Design review of the part built by this model. Coordinates are the model's own, in mm. Coordinates: 2 decimals unless noted, no trailing zeros. Write each loop counter-clockwise with the first axis right and the second up, starting at its lowest first coordinate (ties: lowest second). Pieces come first, ordered by that corner, then holes. Notation, with made-up numbers: (61, -33) - (103, -33) arc R23 ccw to (103, -6) - close; hole circle Ø3 at (-25, 39.5). An arc over 180 degrees is marked (long way). Use a Markdown table: item, result.
from build123d import *

# Parameters (mm, degrees)
SKETCH1_W           = 25.4
SKETCH1_H           = 50.8
SKETCH1_W_2         = 20.32
SKETCH1_H_2         = 45.72
BOSS_EXTRUDE1_DEPTH = 1314.45
SKETCH2_W           = 25.4
SKETCH2_H           = 50.8
BOSS_EXTRUDE2_DEPTH = 6.35
SKETCH3_W           = 25.4
SKETCH3_H           = 50.8
BOSS_EXTRUDE3_DEPTH = 6.35
SKETCH4_W           = 19.05
SKETCH4_H           = 19.05
SKETCH4_W_2         = 12.7
SKETCH4_H_2         = 12.7
BOSS_EXTRUDE4_DEPTH = 558.8


with BuildPart() as part:
    # Sketch1 → Boss-Extrude1 (new body, symmetric)
    with BuildSketch(Plane(origin=(0, 0, 0), x_dir=(0, 0, -1), z_dir=(1, 0, 0))):
        Rectangle(SKETCH1_W, SKETCH1_H)
        Rectangle(SKETCH1_W_2, SKETCH1_H_2, mode=Mode.SUBTRACT)
    extrude(amount=BOSS_EXTRUDE1_DEPTH, both=True)

    # Sketch2 → Boss-Extrude2 (add)
    with BuildSketch(Plane(origin=(1314.45, 0, 0), x_dir=(0, 0, -1), z_dir=(1, 0, 0))):
        Rectangle(SKETCH2_W, SKETCH2_H)
    extrude(amount=BOSS_EXTRUDE2_DEPTH)

    # Sketch3 → Boss-Extrude3 (add)
    with BuildSketch(Plane.ZY.offset(1314.45)):
        Rectangle(SKETCH3_W, SKETCH3_H)
    extrude(amount=BOSS_EXTRUDE3_DEPTH)

    # Sketch4 → Boss-Extrude4 (add)
    with BuildSketch(Plane(origin=(0, 0, -12.7), x_dir=(-1, 0, 0), z_dir=(0, 0, -1))):
        with Locations((-1282.573, -12.7)):
            Rectangle(SKETCH4_W, SKETCH4_H)
        with Locations((-1282.573, -12.7)):
            Rectangle(SKETCH4_W_2, SKETCH4_H_2, mode=Mode.SUBTRACT)
        with Locations((-508, -12.7)):
            Rectangle(SKETCH4_W, SKETCH4_H)
        with Locations((-508, -12.7)):
            Rectangle(SKETCH4_W_2, SKETCH4_H_2, mode=Mode.SUBTRACT)
        with Locations((1282.573, -12.7)):
            Rectangle(SKETCH4_W, SKETCH4_H)
        with Locations((1282.573, -12.7)):
            Rectangle(SKETCH4_W_2, SKETCH4_H_2, mode=Mode.SUBTRACT)
        with Locations((508, -12.7)):
            Rectangle(SKETCH4_W, SKETCH4_H)
        with Locations((508, -12.7)):
            Rectangle(SKETCH4_W_2, SKETCH4_H_2, mode=Mode.SUBTRACT)
    extrude(amount=BOSS_EXTRUDE4_DEPTH)


solid = part.part
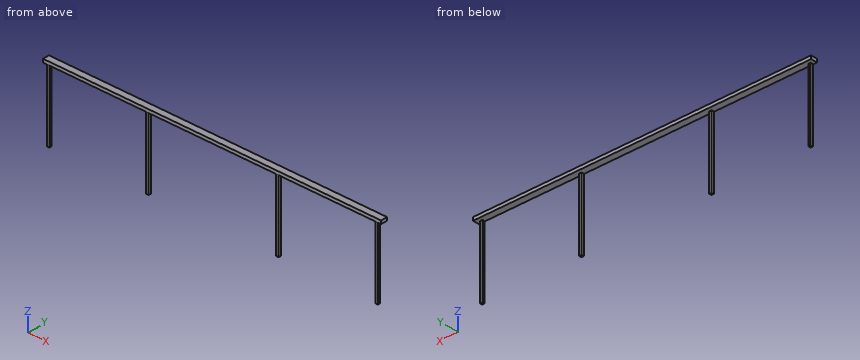
(1) Take a section at C-C on y = 12. Write out the cut boundary in (x, z), and give its area (3 significant figures).
Determined:
| item | result |
|---|---|
| outline | (-1320.8, -12.7) - (1320.8, -12.7) - (1320.8, 12.7) - (-1320.8, 12.7) - close; hole (-1314.45, -10.16) - (1314.45, -10.16) - (1314.45, 10.16) - (-1314.45, 10.16) - close |
| area | 13,700 mm2 |
(2) Take a section at B-B on x = 723. Write out the cut boundary in (y, z).
Determined:
| item | result |
|---|---|
| outline | (-25.4, -12.7) - (25.4, -12.7) - (25.4, 12.7) - (-25.4, 12.7) - close; hole (-22.86, -10.16) - (22.86, -10.16) - (22.86, 10.16) - (-22.86, 10.16) - close |
(3) Take a section at A-A on z = -458. State how many separate pieces and enclosed holes the cut face has, and give its area (3 significant figures).
Determined:
| item | result |
|---|---|
| separate pieces | 4 |
| enclosed holes | 4 |
| area | 806 mm2 |
(4) For L1, parallel to X at y = -20.5, z = -15 (3 decimals); L2, parallel to Z at x = 145, y = 13, list the stretches that pass through material, from the lowest coordinate up. Write a range as from..to.
Determined:
| item | result |
|---|---|
| L1 | -1292.098..-1273.048, -517.525..-498.475, 498.475..517.525, 1273.048..1292.098 |
| L2 | -12.7..-10.16, 10.16..12.7 |
(5) For pin 1 (9.5 mm diameter, centred on x = 1284.5, z = -248, fed in from -Y) (3 decimals); pin 2 (4 mm diameter, centred on x = -1283.5, y = -10.5, fed in from -Z); pin 3 (8 mm diameter, centred on y = 0, z = -99.5, fed in from -X), all flat-tipped, find the tip position at first contact; note any pin that passes through.
Determined:
| item | result |
|---|---|
| pin 1 | y = -22.225 |
| pin 2 | z = -12.7 |
| pin 3 | x = -1292.1 |
